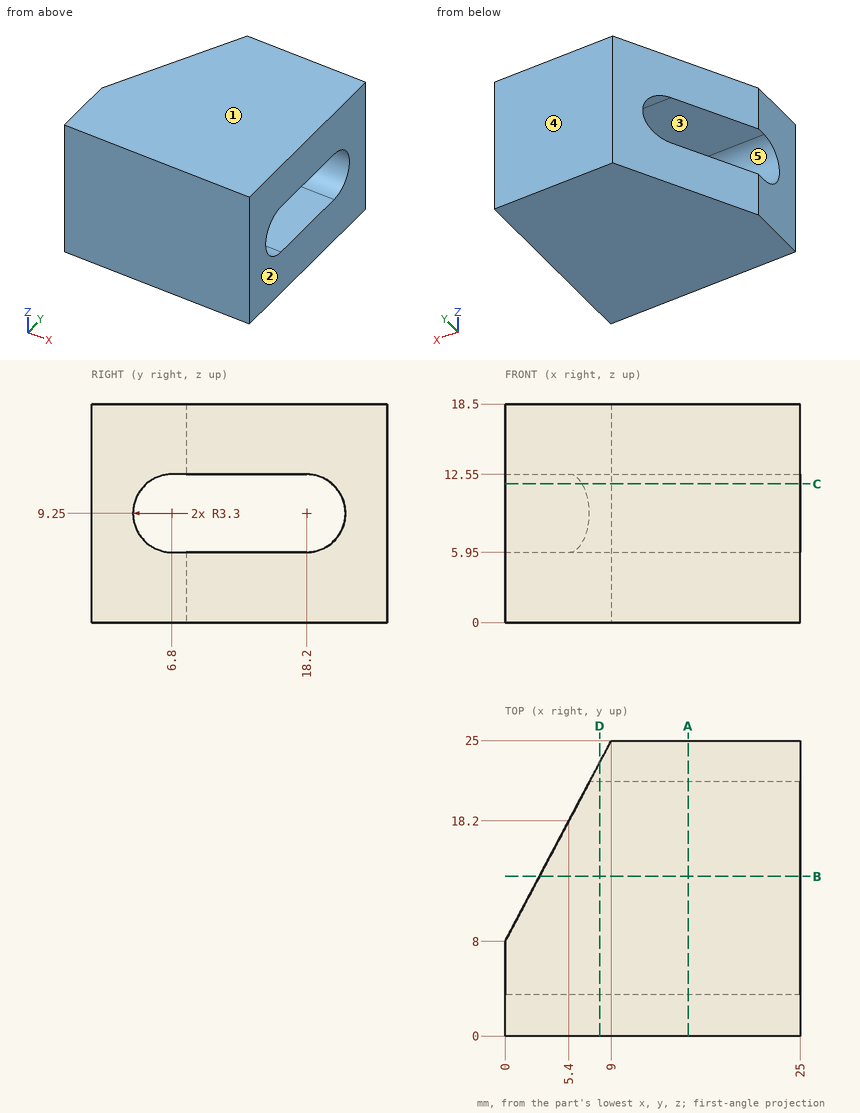
Geometry: see drawing. Coordinates: mm, zero at the bounding-box minimum. A direction names the side the tool comes from. Give positions to 0.01 mm unless a question says otherwise; leave off trailing zeros. Write each loop counter-clockwise with the first axis right and the second up, starting at its lowest first coordinate (ties: lowest second). Pieces come first, ordered by that corner, then holes. Notation, with made-up numbers: (52.25, 28) - (100.25, 28) arc R13 ccw to (100.25, 34) - close; hole circle Ø8 at (-34.75, 7.25). An arc over 180 degrees is marked (long way). Return JSON: item names as keys, results as strings. Group by question number.
1) Set-up query: the marked faces 4 and 5. Return all of +Z, -Z, +X, -X, +Y, -Y with unobstructed straight access to the full face (end or side cutting, diameter ignored); none if empty.
2) Section A-A on x = 15.5. Return the cut outline in (y, z).
3) Line query: line 1 (Z direction, x = 8.5, y = 16.25); line 2 (Y direction, x = 17.25, z = 11.5). Output: solid intervals per line, ascending.
4) Section B-B on y = 13.5. Return the cut outline in (x, z).
5) First-contact query: P1, Ø9, axis at x = 8.5, y = 11, coming from the -Z side; P2, Ø4, axis at y = 17.5, z = 2.5, coming from the -X side. Flat tips, straight axial feed; report the tip coordinate or a pass-through.
6) Section D-D on x = 8. Return the cut outline in (y, z).
7) Mould query, pull axis Z, two halves, no side actions, for the marked faces 1, 2 and 3. Classes: released by +Z, released by -Z, zero draft, split by the parting line, or undercut.
8) Section C-C on z = 11.75. Return the cut outline in (x, y).
Filled in:
{
 "1": {"face 4": "+Z, -Z, +X, -X, +Y", "face 5": "+X, -X"},
 "2": {"outline": "(0, 0) - (25, 0) - (25, 18.5) - (0, 18.5) - close; hole (6.8, 5.95) - (18.2, 5.95) arc R3.3 ccw to (18.2, 12.55) - (6.8, 12.55) arc R3.3 ccw to start"},
 "3": {"line 1": "z = 0 to 5.95, 12.55 to 18.5", "line 2": "y = 0 to 4.39, 20.61 to 25"},
 "4": {"outline": "(2.91, 0) - (25, 0) - (25, 5.95) - (2.91, 5.95) - close; (2.91, 12.55) - (25, 12.55) - (25, 18.5) - (2.91, 18.5) - close"},
 "5": {"P1": "stops at z = 0", "P2": "stops at x = 3.97"},
 "6": {"outline": "(0, 0) - (23.11, 0) - (23.11, 18.5) - (0, 18.5) - close; hole (6.8, 5.95) - (18.2, 5.95) arc R3.3 ccw to (18.2, 12.55) - (6.8, 12.55) arc R3.3 ccw to start"},
 "7": {"face 1": "released by +Z", "face 2": "zero draft", "face 3": "undercut"},
 "8": {"outline": "(0, 0) - (25, 0) - (25, 4.65) - (0, 4.65) - close; (6.54, 20.35) - (25, 20.35) - (25, 25) - (9, 25) - close"}
}
